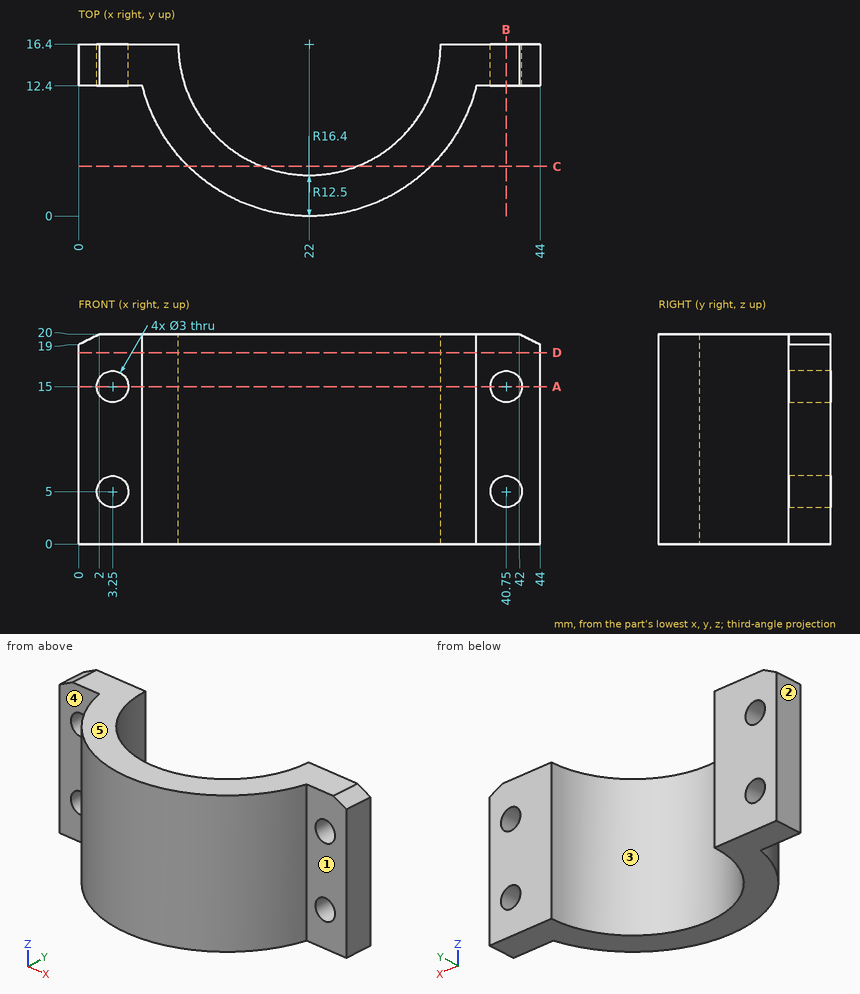
For this review, use the dimensioned drawing (mm, ordinates from the lowest corner) and the shaded views. A direction names the side the tool comes from. Give positions to 0.01 mm unless a question says otherwise; leave off trailing zeros. Write each loop counter-clockwise with the first axis right and the second up, starting at its lowest first coordinate (ties: lowest second). Pieces come first, ordered by that corner, then holes.
(1) Tool access review of the marked faces 4 and 5: name each direction out of +Z, -Z, +X, -X, +Y, -Y from which nothing blocks a thin tool from reaching the whole face with its end or side.
(2) Consider section D-D, the plane z = 18.25. Give the boundary of the cut face in (x, y), and give its area (3 significant figures).
(3) Consider section A-A, the plane z = 15. Give the boundary of the cut face in (x, y), and give its area (3 significant figures).
(4) The part is to be moulded in two halves that separate along X. For the marked faces 1, 2 and 3, say which applies: released by +X, released by -X, zero draft, split by the parting line, or undercut.
(5) Consider section C-C, the plane y = 4.75. Give the boundary of the cut face in (x, z).
(6) For P1, Ø3, axis at x = 40, z = 5.5, coming from the -Y side; P2, Ø8, axis at y = 4.5, z = 10.5, coming from the -X side; P3, Ø5, axis at x = 38.5, z = 11, coming from the -Y side; P4, Ø3, axis at x = 8.5, y = 11, coming from the -Z side, all flat-tipped, find the tip position at first contact; note any pin that passes through.
(7) To check wall thickness, follow L1, parallel to X at y = 15.15, z = 5; L2, parallel to Z at x = 2, y = 12.75; L3, parallel to X at y = 12.5, z = 16. State the ranges of each line that lie inside material, in increasing order.
(8) Consider section B-B, the plane x = 40.75. Give the boundary of the cut face in (y, z), and give its area (3 significant figures).
Returned:
1. face 4: +Z, -Z, -X, -Y
1. face 5: +Z, +X, -X, +Y, -Y
2. outline: (0, 12.4) - (6.1, 12.4) arc R16.4 ccw to (37.9, 12.4) - (44, 12.4) - (44, 16.4) - (34.5, 16.4) arc R12.5 cw to (9.5, 16.4) - (0, 16.4) - close
2. area: 223 mm2
3. outline: (0, 12.4) - (1.75, 12.4) - (1.75, 16.4) - (0, 16.4) - close; (4.75, 12.4) - (6.1, 12.4) arc R16.4 ccw to (37.9, 12.4) - (39.25, 12.4) - (39.25, 16.4) - (34.5, 16.4) arc R12.5 cw to (9.5, 16.4) - (4.75, 16.4) - close; (42.25, 12.4) - (44, 12.4) - (44, 16.4) - (42.25, 16.4) - close
3. area: 199 mm2
4. face 1: zero draft
4. face 2: released by -X
4. face 3: undercut
5. outline: (10.46, 0) - (17.47, 0) - (17.47, 20) - (10.46, 20) - close; (26.53, 0) - (33.54, 0) - (33.54, 20) - (26.53, 20) - close
6. P1: stops at y = 12.4
6. P2: stops at x = 7.63
6. P3: stops at y = 7.86
6. P4: stops at z = 0
7. L1: x = 0 to 1.75, 4.75 to 9.56, 34.44 to 39.25, 42.25 to 44
7. L2: z = 0 to 4.17, 5.83 to 14.17, 15.83 to 20
7. L3: x = 0 to 2.13, 4.37 to 10.12, 33.88 to 39.63, 41.87 to 44
8. outline: (12.4, 0) - (16.4, 0) - (16.4, 3.5) - (12.4, 3.5) - close; (12.4, 6.5) - (16.4, 6.5) - (16.4, 13.5) - (12.4, 13.5) - close; (12.4, 16.5) - (16.4, 16.5) - (16.4, 20) - (12.4, 20) - close
8. area: 56.0 mm2
